```python
from build123d import *

# Parameters (mm, degrees)
SKETCH1_R           = 1.5
BOSS_EXTRUDE1_DEPTH = 3


with BuildPart() as part:
    # Sketch1 → Boss-Extrude1 (new body)
    with BuildSketch(Plane(origin=(0, 0, 0), x_dir=(1, 0, 0), z_dir=(0, 1, 0))):
        with BuildLine():
            Line((-2, 83), (2, 83))
            Line((2, 83), (4.494360181, 33.225225593))
            ThreePointArc((4.494360181, 33.225225593), (4.457597858, 32.38370353), (4.264652125, 31.563775))
            Line((4.264652125, 31.563775), (15.063775, 20.764652125))
            ThreePointArc((15.063775, 20.764652125), (21, 16.5), (15.063775, 12.235347875))
            Line((15.063775, 12.235347875), (4.264652125, 1.436225))
            ThreePointArc((4.264652125, 1.436225), (0, -4.5), (-4.264652125, 1.436225))
            Line((-4.264652125, 1.436225), (-15.063775, 12.235347875))
            ThreePointArc((-15.063775, 12.235347875), (-21, 16.5), (-15.063775, 20.764652125))
            Line((-15.063775, 20.764652125), (-4.264652125, 31.563775))
            ThreePointArc((-4.264652125, 31.563775), (-4.454454203, 32.361378239), (-4.496391332, 33.180180433))
            Line((-4.496391332, 33.180180433), (-2, 83))
        make_face()
        Circle(SKETCH1_R, mode=Mode.SUBTRACT)
        with Locations((0, 33)):
            Circle(SKETCH1_R, mode=Mode.SUBTRACT)
        with Locations((-16.5, 16.5)):
            Circle(SKETCH1_R, mode=Mode.SUBTRACT)
        with Locations((16.5, 16.5)):
            Circle(SKETCH1_R, mode=Mode.SUBTRACT)
        with BuildLine():
            Line((12.235347875, 17.936225), (1.436225, 28.735347875))
            ThreePointArc((1.436225, 28.735347875), (0, 28.5), (-1.436225, 28.735347875))
            Line((-1.436225, 28.735347875), (-12.235347875, 17.936225))
            ThreePointArc((-12.235347875, 17.936225), (-12, 16.5), (-12.235347875, 15.063775))
            Line((-12.235347875, 15.063775), (-1.436225, 4.264652125))
            ThreePointArc((-1.436225, 4.264652125), (0, 4.5), (1.436225, 4.264652125))
            Line((1.436225, 4.264652125), (12.235347875, 15.063775))
            ThreePointArc((12.235347875, 15.063775), (12, 16.5), (12.235347875, 17.936225))
        make_face(mode=Mode.SUBTRACT)
    extrude(amount=BOSS_EXTRUDE1_DEPTH)


solid = part.part
```
Source: CAD feature listing. Evaluate the final solid. Frame: model axes, mm. A direction names the side the tool comes from. Give positions to 0.01 mm unless a question says otherwise; leave off trailing zeros. Write each loop counter-clockwise with the first axis right and the second up, starting at its lowest first coordinate (ties: lowest second). Pieces come first, ordered by that corner, then holes.
1. Access query for faces 4 (the face through (-6.76, 1.48, -23.41)), 5 (the face through (-3.266, 1.479, -57.741)). Directions: +Z, -Z, +X, -X, +Y, -Y. A direction counts if a zero-diameter tool reaches every point of the face in a straight line with its end or side. Return the directions, or none.
2. Section query A-A (z = -16.5). Return the cut outline in (x, y).
3. First-contact query: pin 1 (1.8 mm diameter, centred on x = 0, z = -33, fed in from -Y); pin 2 (3 mm diameter, centred on x = 4.5, z = -59.5, fed in from +Y); pin 3 (1 mm diameter, centred on x = -8.5, y = 1.5, fed in from +Z); pin 4 (1.5 mm diameter, centred on x = -13, y = 1, fed in from +Z). Flat tips, straight axial feed; report the tip coordinate or a pass-through.
4. Section query B-B (z = 0). Return the cut outline in (x, y), then the cut area to 3 significant figures.
5. Section query C-C (x = 16.5). Return the cut outline in (y, z), then the cut area to 3 significant figures.
6. Section query D-D (y = 0.45). Return the cut outline in (x, z).
7. Material intervals for line 1 along X through (y, z) = (1.5, -16.5); line 2 along X through (y, z) = (1.85, 0); line 3 along Z through (x, y) = (-16.5, 1.9), sorted ascending.
8. Pull-direction query (Z, two-part tool) for faces 1 (the face through (2, 3, -30)), 2 (the face through (0, 1.5, -4.5)), 3 (the face through (0, 1, -83)); classes: +Z half, -Z half, draft (parallel to the pull), parting line (faces both ways), or undercut.
Output values:
1. face 4: +Y, -Y
1. face 5: -Z, -X, +Y, -Y
2. outline: (-21, 0) - (-18, 0) - (-18, 3) - (-21, 3) - close; (-15, 0) - (-12, 0) - (-12, 3) - (-15, 3) - close; (12, 0) - (15, 0) - (15, 3) - (12, 3) - close; (18, 0) - (21, 0) - (21, 3) - (18, 3) - close
3. pin 1: passes through
3. pin 2: stops at y = 3
3. pin 3: stops at z = -5.17
3. pin 4: stops at z = -9.42
4. outline: (-4.5, 0) - (-1.5, 0) - (-1.5, 3) - (-4.5, 3) - close; (1.5, 0) - (4.5, 0) - (4.5, 3) - (1.5, 3) - close
4. area: 18.0 mm2
5. outline: (0, -21) - (3, -21) - (3, -18) - (0, -18) - close; (0, -15) - (3, -15) - (3, -12) - (0, -12) - close
5. area: 18.0 mm2
6. outline: (-15.06, -20.76) - (-4.26, -31.56) arc R4.5 ccw to (-4.5, -33.18) - (-2, -83) - (2, -83) - (4.49, -33.23) arc R4.5 ccw to (4.26, -31.56) - (15.06, -20.76) arc R4.5 ccw (long way) to (15.06, -12.24) - (4.26, -1.44) arc R4.5 ccw (long way) to (-4.26, -1.44) - (-15.06, -12.24) arc R4.5 ccw (long way) to start; hole circle Ø3 at (-16.5, -16.5); hole (-12.24, -17.94) - (-1.44, -28.74) arc R4.5 cw to (1.44, -28.74) - (12.24, -17.94) arc R4.5 cw to (12.24, -15.06) - (1.44, -4.26) arc R4.5 cw to (-1.44, -4.26) - (-12.24, -15.06) arc R4.5 cw to start; hole circle Ø3 at (0, -33); hole circle Ø3 at (0, 0); hole circle Ø3 at (16.5, -16.5)
7. line 1: x = -21 to -18, -15 to -12, 12 to 15, 18 to 21
7. line 2: x = -4.5 to -1.5, 1.5 to 4.5
7. line 3: z = -21 to -18, -15 to -12
8. face 1: draft
8. face 2: undercut
8. face 3: -Z half
